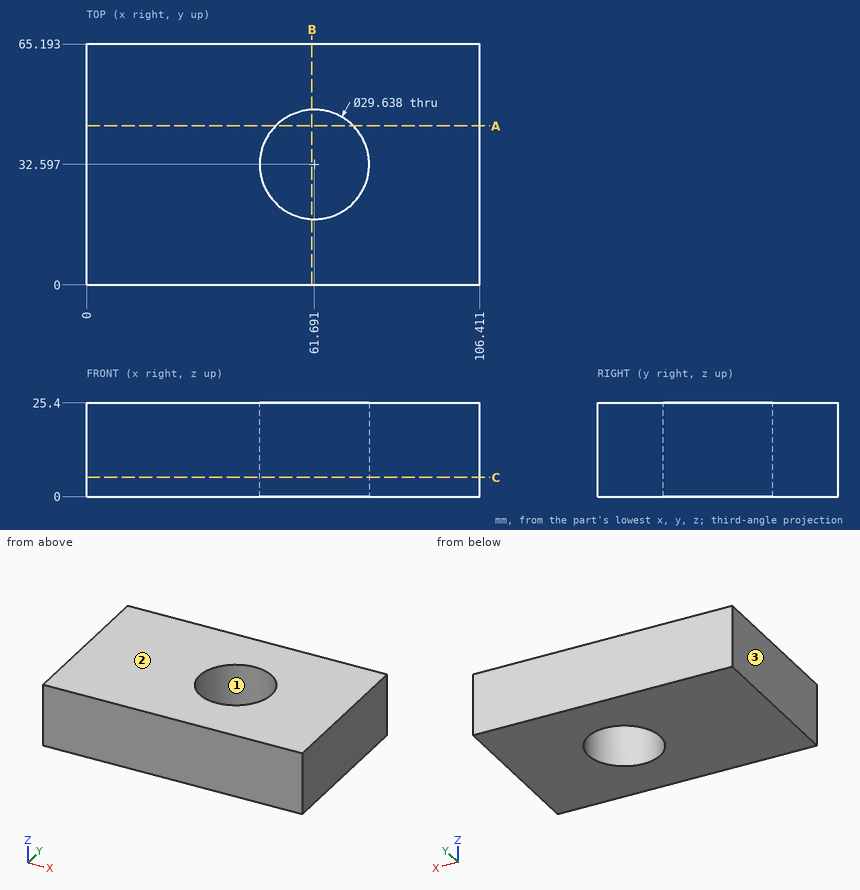
Geometry check sheet. Reference: drawing and pictorial views, mm from the part's lowest x, y, z. Give positions to 0.01 mm unless a question says otherwise; leave off trailing zeros. Order: outer loops, then holes, each group sorted by start corner. A loop starts at its lowest first (then second) coordinate and runs counter-clockwise, first axis right, second up. Notation, with made-up numbers: M -1,-22 L 56,-22 A28 cw 56,17 Z; hole C -38.75,-8.75 d9. An arc over 180 degrees is marked long. Answer as CSV lines item,"result". Start each with the question number.
Item 1: Cross-section at C-C on z = 5.25. Enter the section's corners in (x, y).
Item 2: Cross-section at A-A on y = 43. Enter the section's corners in (x, z) (1 decimal), plus the area to 3 significant figures.
Item 3: Thickness scan on line 1 (Y direction, x = 51, z = 6.25) (1 decimal); line 2 (X direction, y = 41, z = 5.75) (1 decimal); line 3 (Y direction, x = 53, z = 8) (1 decimal). Record the ranges inside material, lowest first. Write a range as [from, to].
Item 4: Mould release check, pull along X, two halves, no side actions. Record for the marked faces 1, 2 and 3: +X half, -X half, draft (parallel to the pull), parting line (faces both ways), or undercut.
Item 5: Gauge pin test, flat end, axial feed: P1, Ø5, axis at x = 40, y = 8.5, coming from the -Z side. Record the tip position at first contact, or that the pin passes through.
Item 6: Cross-section at B-B on x = 61. Enter the section's corners in (y, z).
Established:
1,outline,"M 0,0 L 106.41,0 L 106.41,65.19 L 0,65.19 Z; hole C 61.69,32.6 d29.64"
2,outline,"M 0,0 L 51.1,0 L 51.1,25.4 L 0,25.4 Z; M 72.2,0 L 106.4,0 L 106.4,25.4 L 72.2,25.4 Z"
2,area,"2,170 mm^2"
3,line 1,"y = [0, 22.3], [42.9, 65.2]"
3,line 2,"x = [0, 49.5], [73.9, 106.4]"
3,line 3,"y = [0, 20.6], [44.6, 65.2]"
4,face 1,"undercut"
4,face 2,"draft"
4,face 3,"-X half"
5,P1,"stops at z = 0"
6,outline,"M 0,0 L 17.79,0 L 17.79,25.4 L 0,25.4 Z; M 47.4,0 L 65.19,0 L 65.19,25.4 L 47.4,25.4 Z"
